Study the drawing (mm; zero at the part's minimum x, y, z) and answer. Round coordinates to 2 decimals unless told otherwise and drop trailing zeros. Write each loop counter-clockwise with the first axis right and the second up, starting at its lowest first coordinate (ties: lowest second). Pieces come first, ordered by that corner, then holes. Notation, with made-up numbers: (-40, 72.25) - (-36, 72.25) arc R5 ccw to (-36, 77.25) - close; hole circle Ø9 at (-38, 3.5). An arc over 180 degrees is marked (long way). Return JSON: item names as keys, results as strings. Group by question number.
(1) Determine the mould class of the marked faces 1, 2, 3 and 4 for opening direction X: +X half, -X half, draft (parallel to the pull), parting line (faces both ways), or undercut.
(2) Find the intervals of material crossed by line 1 along Y through (x, z) = (25.4, 12) (3 decimals); line 2 along Y through (x, z) = (23.5, 9.25); line 3 along Z through (x, y) = (20, 5.5), in increasing order. Write a range as [from, to].
(3) Each of these flat-tipped pins is pushed along its axis until it touches: pin 1 (10 mm diameter, centred on y = 41, z = 8.5, fed in from -X); pin 2 (12 mm diameter, centred on x = 16.5, z = 11, fed in from -Y); pin 3 (5.5 mm diameter, centred on x = 25.4, y = 44.45, fed in from +Z); pin 4 (12 mm diameter, centred on x = 24, z = 5.5, fed in from -Y). Where does it stop, or does it pass through?
(4) Section A-A, the plane z = 19 is taken. Write down the section's boundary in (x, y) (3 decimals), then the cut area to 3 significant figures.
(5) Section B-B, the plane x = 25.4 is taken. Give the number of separate pieces and of enclosed holes in the cut face, then the cut area to 3 significant figures.
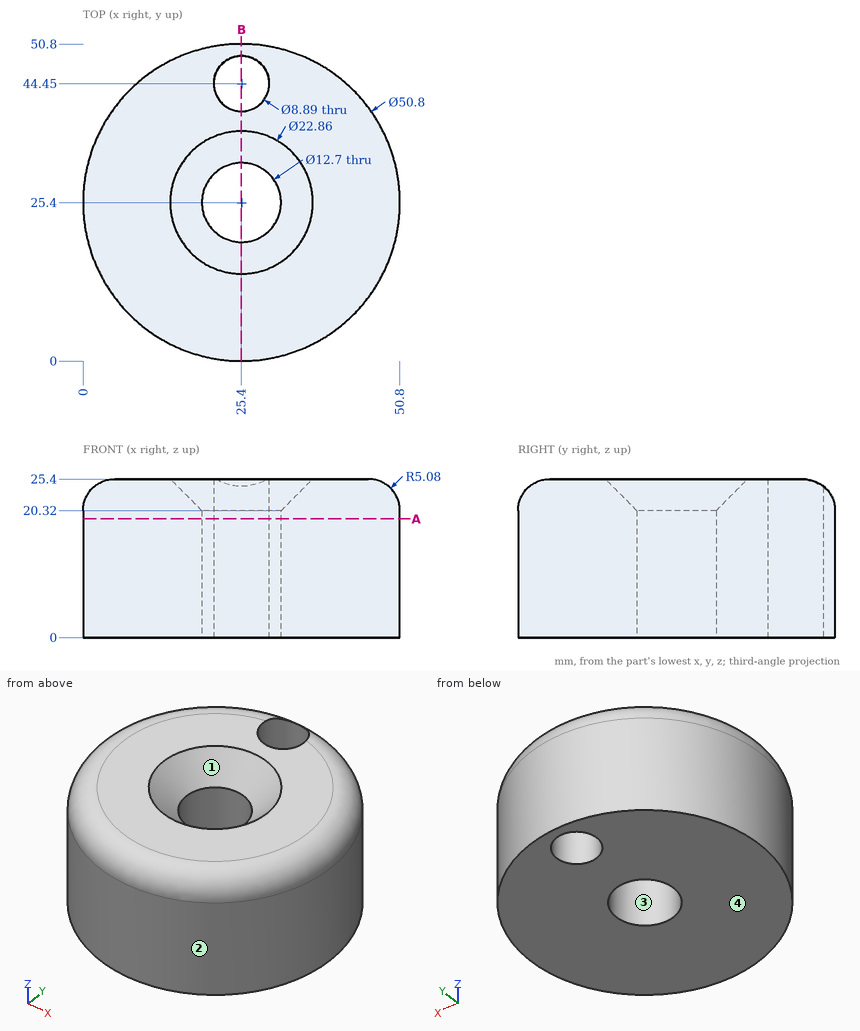
Working result:
{
 "1": {"face 1": "undercut", "face 2": "parting line", "face 3": "undercut", "face 4": "draft"},
 "2": {"line 1": "y = [0, 19.05], [31.75, 40.005], [48.895, 50.8]", "line 2": "y = [0.07, 19.34], [31.46, 40.43], [48.47, 50.73]", "line 3": "z = [0, 25.39]"},
 "3": {"pin 1": "stops at x = 2.32", "pin 2": "stops at y = 0.17", "pin 3": "passes through", "pin 4": "stops at y = 0"},
 "4": {"outline": "circle Ø50.8 at (25.4, 25.4); hole circle Ø12.7 at (25.4, 25.4); hole circle Ø8.89 at (25.4, 44.45)", "area": "1,840 mm^2"},
 "5": {"separate pieces": "3", "enclosed holes": "0", "area": "706 mm^2"}
}
